```python
from build123d import *

# Parameters (mm, degrees)
BOSS_EXTRU_1_DEPTH      = 10
ESQUISSE2_W             = 10
ESQUISSE2_H             = 10
BOSS_EXTRU_2_DEPTH      = 15
ESQUISSE3_W             = 10
ESQUISSE3_H             = 10
BOSS_EXTRU_3_DEPTH      = 15
ESQUISSE4_R             = 2
ENL_V_MAT_EXTRU_1_DEPTH = 20


with BuildPart() as part:
    # Esquisse1 → Boss.-Extru.1 (new body)
    with BuildSketch(Plane.XY):
        with BuildLine():
            Line((-22.399928161, 17.075), (-17.399928161, 17.075))
            ThreePointArc((-17.399928161, 17.075), (0, -0.375), (17.399928161, 17.075))
            Line((17.399928161, 17.075), (22.399928161, 17.075))
            Line((22.399928161, 17.075), (22.399928161, -17.075))
            Line((22.399928161, -17.075), (-22.399928161, -17.075))
            Line((-22.399928161, -17.075), (-22.399928161, 17.075))
        make_face()
    extrude(amount=BOSS_EXTRU_1_DEPTH)

    # Esquisse2 → Boss.-Extru.2 (add)
    with BuildSketch(Plane.ZY.offset(22.399928161)):
        with Locations((5, -12.075)):
            Rectangle(ESQUISSE2_W, ESQUISSE2_H)
    extrude(amount=BOSS_EXTRU_2_DEPTH)

    # Esquisse3 → Boss.-Extru.3 (add)
    with BuildSketch(Plane(origin=(22.399928161, 0, 0), x_dir=(0, 0, -1), z_dir=(1, 0, 0))):
        with Locations((-5, -12.075)):
            Rectangle(ESQUISSE3_W, ESQUISSE3_H)
    extrude(amount=BOSS_EXTRU_3_DEPTH)

    # Esquisse4 → Enlèv. mat.-Extru.1 (cut)
    with BuildSketch(Plane(origin=(0, -7.075, 0), x_dir=(1, 0, 0), z_dir=(0, 1, 0))):
        with Locations(Location((-30.399928161, -5, 0), (0, 0, 180))):
            Circle(ESQUISSE4_R)
        with Locations(Location((30.399928161, -5, 0), (0, 0, 270))):
            Circle(ESQUISSE4_R)
    extrude(amount=-ENL_V_MAT_EXTRU_1_DEPTH, mode=Mode.SUBTRACT)


solid = part.part
```
Geometry check sheet. Reference: the model listing, model coordinates, mm. A direction names the side the tool comes from. Round coordinates to 2 decimals unless told otherwise and drop trailing zeros. Order: outer loops, then holes, each group sorted by start corner. A loop starts at its lowest first (then second) coordinate and runs counter-clockwise, first axis right, second up. Notation, with made-up numbers: (-25.75, 88) - (-21.75, 88) arc R29 cw to (-21.75, 112) - close; hole circle Ø2 at (77.5, 8.25). An arc over 180 degrees is marked (long way). Use a Markdown table: item, result. Add a question column.
(1) Material ranges on line 1 along X through (y, z) = (-9.5, 6.5); line 2 along Y through (x, z) = (23, 9) (3 decimals); line 3 along X through (y, z) = (5, 7), recorded low to high. Write a range as [from, to].
(2) Sectioned sample at D-D, the plane x = 0. Enter the section's corners in (y, z) (3 decimals), and give its area (3 significant figures).
(3) Sectioned sample at C-C, the plane y = 11.5. Enter the section's corners in (x, z).
(4) Tool access check on faces 5 (the flat face through (22.4, 5, 5)), 6 (the flat face through (-22.4, 5, 5)), 7 (the flat face through (-37.4, -12, 5)). Record the directions out of +Z, -Z, +X, -X, +Y, -Y that give a thin tool (end or side, any length) a straight path to the whole face; none if there is none.
(5) Sectioned sample at B-B, the plane x = 29.5. Enter the section's corners in (y, z) (3 decimals), and give its area (3 significant figures).
(6) Release check for a two-part mould opening along Z. For faces 1 (the cylindrical face through (-28.4, -12, 5.09)), 2 (the cylindrical face through (-0.38, -0.37, 4.93)), 3 (the cylindrical face through (32.383, -12.005, 4.74)), 4 (the flat face through (-1, -8, 10)) record: pulls with the +Z half, pulls with the -Z half, needs draft (parallel to the pull), parting line crosses it, or undercut.
(7) Depth check by flat-ended pin: pin 1 (5 mm diameter, centred on x = -27.5, z = 4, fed in from +Y) (3 decimals); pin 2 (2 mm diameter, centred on y = -4, z = 3, fed in from +X); pin 3 (1.5 mm diameter, centred on y = 6.5, z = 7.5, fed in from -X). Enter the tip coordinate at first touch or a pass-through.
(8) Sectioned sample at A-A, the plane z = 5. Enter the section's corners in (x, y) (3 decimals).
Answers below:
| question | item | result |
|---|---|---|
| 1 | line 1 | [-37.4, -31.72], [-29.08, 29.08], [31.72, 37.4] |
| 1 | line 2 | [-17.075, -7.075] |
| 1 | line 3 | [-22.4, -12.58], [12.58, 22.4] |
| 2 | outline | (-17.075, 0) - (-0.375, 0) - (-0.375, 10) - (-17.075, 10) - close |
| 2 | area | 167 mm² |
| 3 | outline | (-22.4, 0) - (-16.5, 0) - (-16.5, 10) - (-22.4, 10) - close; (16.5, 0) - (22.4, 0) - (22.4, 10) - (16.5, 10) - close |
| 4 | face 5 | +Z, -Z, +X, +Y |
| 4 | face 6 | +Z, -Z, -X, +Y |
| 4 | face 7 | +Z, -Z, -X, +Y, -Y |
| 5 | outline | (-17.075, 0) - (-7.075, 0) - (-7.075, 3.214) - (-17.075, 3.214) - close; (-17.075, 6.786) - (-7.075, 6.786) - (-7.075, 10) - (-17.075, 10) - close |
| 5 | area | 64.3 mm² |
| 6 | face 1 | undercut |
| 6 | face 2 | needs draft |
| 6 | face 3 | undercut |
| 6 | face 4 | pulls with the +Z half |
| 7 | pin 1 | y = -7.075 |
| 7 | pin 2 | x = 22.4 |
| 7 | pin 3 | x = -22.4 |
| 8 | outline | (-37.4, -17.075) - (-32.4, -17.075) - (-32.4, -7.075) - (-37.4, -7.075) - close; (-28.4, -17.075) - (28.4, -17.075) - (28.4, -7.075) - (22.4, -7.075) - (22.4, 17.075) - (17.4, 17.075) arc R17.4 cw (long way) to (-17.4, 17.075) - (-22.4, 17.075) - (-22.4, -7.075) - (-28.4, -7.075) - close; (32.4, -17.075) - (37.4, -17.075) - (37.4, -7.075) - (32.4, -7.075) - close |
